CAD build for the part. Positions are in the model's coordinates, mm. A direction names the side the tool comes from. Coordinates: 2 decimals unless noted, no trailing zeros. Loops run counter-clockwise (first coordinate to the right, second up) from the corner with the lowest first, then second, coordinate; pieces in that order, holes last. Notation, with made-up numbers: (20, 69) -> (70, 69) arc R16 cw to (70, 79) -> close; hole circle Ø10 at (-23, 1). An arc over 180 degrees is marked (long way). Write each question's results on one line, items separated by ' | '.
from build123d import *

# Parameters (mm, degrees)
EXTRUDE_THIN1_DEPTH = 46.75
CHAMFER1_SIZE       = 1
CUT_EXTRUDE1_DEPTH  = 10


with BuildPart() as part:
    # Sketch1 → Extrude-Thin1 (new, symmetric)
    with BuildSketch(Plane.XY):
        Polygon((10, 0), (0, 0), (0, 7), (1.8, 7), (1.8, 1.8), (10, 1.8), align=None)
    extrude(amount=EXTRUDE_THIN1_DEPTH, both=True)

    # Chamfer1
    chamfer1_edges = [part.edges().sort_by_distance(p)[0] for p in [
        (10, 1.8, 0),
    ]]
    chamfer(chamfer1_edges, length=CHAMFER1_SIZE)

    # Sketch2 → Cut-Extrude1 (cut)
    with BuildSketch(Plane(origin=(0, 1.8, 0), x_dir=(1, 0, 0), z_dir=(0, 1, 0))):
        with BuildLine():
            Line((11.522549571, -44.75), (3.9, -44.75))
            ThreePointArc((3.9, -44.75), (2.8, -43.65), (3.9, -42.55))
            Line((3.9, -42.55), (11.522549571, -42.55))
            ThreePointArc((11.522549571, -42.55), (12.622549571, -43.65), (11.522549571, -44.75))
        make_face()
    cut_extrude1 = extrude(amount=-CUT_EXTRUDE1_DEPTH, mode=Mode.SUBTRACT)

    # Mirror1: Cut-Extrude1 across plane
    add(cut_extrude1.mirror(Plane.XY), mode=Mode.SUBTRACT)


solid = part.part
1) Slice it at A-A (x = 5). Write the cut outline in (y, z).
Outcome:
outline: (0, -46.75) -> (1.8, -46.75) -> (1.8, -44.75) -> (0, -44.75) -> close; (0, -42.55) -> (1.8, -42.55) -> (1.8, 42.55) -> (0, 42.55) -> close; (0, 44.75) -> (1.8, 44.75) -> (1.8, 46.75) -> (0, 46.75) -> close
2) Two-plate mould, pull along Z, no slides. Class faces 4 (the flat face through (7, 1, 42.55)), 5 (the flat face through (1, 7, 1)), 6 (the flat face through (3, 1, 46.75)): pulls with the +Z half, pulls with the -Z half, needs draft (parallel to the pull), parting line crosses it, or undercut.
Outcome:
face 4: undercut | face 5: needs draft | face 6: pulls with the +Z half
3) Which spindle directions (+Z, -Z, +X, -X, +Y, -Y) get a long thin tool onto all of the face, cutting with end or side? Do faces 1 (the flat face through (5, 1.8, 1)), 2 (the flat face through (7, 1, -44.75)), 3 (the flat face through (0, 3, 1)). Say none if no direction does.
Outcome:
face 1: +Z, -Z, +X, +Y | face 2: +X, +Y, -Y | face 3: +Z, -Z, -X, +Y, -Y
4) Slice it at B-B (z = 4.5). Write the cut outline in (x, y), then the cut area to 3 significant figures.
Outcome:
outline: (0, 0) -> (10, 0) -> (10, 0.8) -> (9, 1.8) -> (1.8, 1.8) -> (1.8, 7) -> (0, 7) -> close | area: 26.9 mm^2
5) Slice it at C-C (y = 3.75). Write the cut outline in (x, z), then the cut area to 3 significant figures.
Outcome:
outline: (0, -46.75) -> (1.8, -46.75) -> (1.8, 46.75) -> (0, 46.75) -> close | area: 168 mm^2
6) Drill centre lines: L1, parallel to Z at x = 6.25, y = 0.75; L2, parallel to Y at x = 5, z = 20.5. Where is each one in solid material? Low to high. Write a range as from..to.
Outcome:
L1: z = -46.75..-44.75, -42.55..42.55, 44.75..46.75 | L2: y = 0..1.8
7) Slice it at D-D (z = -43.65). Write the cut outline in (x, y).
Outcome:
outline: (0, 0) -> (2.8, 0) -> (2.8, 1.8) -> (1.8, 1.8) -> (1.8, 7) -> (0, 7) -> close
8) Pin check, flat tip, straight feed: pin 1 (6 mm diameter, centred on x = 6, z = 1, fed in from +Y). Stop position of the tip, or through.
Outcome:
pin 1: stops at y = 1.8
